Can you work these out from the drawing? Everything is in mm from the part's minimum corner. A direction names the side the tool comes from. Coordinates: 2 decimals unless noted, no trailing zeros. Order: outer loops, then holes, each group sorted by start corner. A loop starts at its lowest first (then second) coordinate and runs counter-clockwise, first axis right, second up. Notation, with made-up numbers: M 41,65 L 54,65 A14 cw 54,83 Z; hole C 89,11 d7. An arc over 180 degrees is marked long. Answer as a JSON object with one key per item and string values.
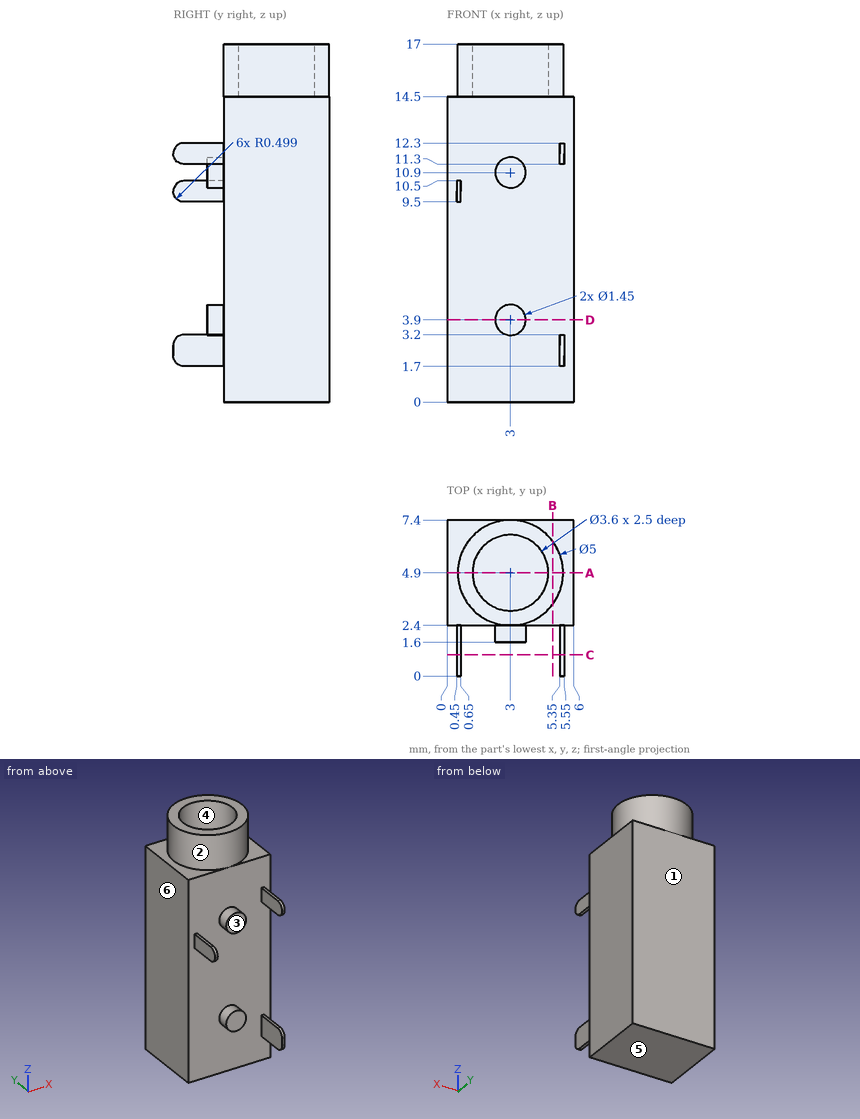
Item 1: Please list where these lines run through material, in increasing order: line 1 (Y direction, x = 3, z = 16); line 2 (Z direction, x = 0.4, y = 4); line 3 (Y direction, x = 0.7, z = 4.25).
Answers follow:
{"line 1": "y = 2.4 to 3.1, 6.7 to 7.4", "line 2": "z = 0 to 14.5", "line 3": "y = 2.4 to 7.4"}
Item 2: I want a section at C-C, the plane y = 1. Write out the boundary of the cut face in (x, z).
Answers follow:
{"outline": "M 0.45,9.5 L 0.65,9.5 L 0.65,10.5 L 0.45,10.5 Z; M 5.35,1.7 L 5.55,1.7 L 5.55,3.2 L 5.35,3.2 Z; M 5.35,11.3 L 5.55,11.3 L 5.55,12.3 L 5.35,12.3 Z"}
Item 3: I'm going to push flat-ended pins straight in: pin 1 (1 mm diameter, centred on x = 0.5, z = 4.5, fed in from -Y); pin 2 (1.8 mm diameter, centred on x = 3, z = 5, fed in from -Y); pin 3 (0.5 mm diameter, centred on y = 1.5, z = 2, fed in from +X). Where does each tip first touch, or does it pass through?
Answers follow:
{"pin 1": "stops at y = 2.4", "pin 2": "stops at y = 1.6", "pin 3": "stops at x = 5.55"}
Item 4: I want a section at B-B, the plane x = 5. Write out the boundary of the cut face in (y, z).
Answers follow:
{"outline": "M 2.4,0 L 7.4,0 L 7.4,14.5 L 6.4,14.5 L 6.4,17 L 3.4,17 L 3.4,14.5 L 2.4,14.5 Z"}
Item 5: I want a section at A-A, the plane y = 4.9. Write out the boundary of the cut face in (x, z).
Answers follow:
{"outline": "M 0,0 L 6,0 L 6,14.5 L 5.5,14.5 L 5.5,17 L 4.8,17 L 4.8,14.5 L 1.2,14.5 L 1.2,17 L 0.5,17 L 0.5,14.5 L 0,14.5 Z"}
Item 6: I want a section at D-D, the plane z = 3.9. Write out the boundary of the cut face in (x, y) (1 decimal).
Answers follow:
{"outline": "M 0,2.4 L 2.3,2.4 L 2.3,1.6 L 3.7,1.6 L 3.7,2.4 L 6,2.4 L 6,7.4 L 0,7.4 Z"}
Item 7: If we mould it in two halves opening along X, with no side actions, what happens to the marked faces 4, 5 and 6? For each: pulls with the +X half, pulls with the -X half, needs draft (parallel to the pull), parting line crosses it, or undercut.
Answers follow:
{"face 4": "undercut", "face 5": "needs draft", "face 6": "pulls with the -X half"}
Item 8: Which directions (+Z, -Z, +X, -X, +Y, -Y) give clear straight access to the entire face, cutting with the end or side of a thin tool? Please do the marked faces 1, 2 and 3.
Answers follow:
{"face 1": "+Z, -Z, +X, -X, +Y", "face 2": "+Z", "face 3": "+Z, -Z, -Y"}
